Check sheet for the modelled part. Datum: model origin and axes. Units: mm. Face numbers are marked on the shaded views. A direction names the side the tool comes from. Coordinates: 2 decimals unless noted, no trailing zeros. Loops run counter-clockwise (first coordinate to the right, second up) from the corner with the lowest first, then second, coordinate; pieces in that order, holes last.
```python
from build123d import *

# Parameters (mm, degrees)
SKETCH1_W           = 46.99
SKETCH1_H           = 15.875
BOSS_EXTRUDE1_DEPTH = 21.59
SKETCH2_W           = 43.18
SKETCH2_H           = 12.7
SKETCH2_W_2         = 27.94
SKETCH2_H_2         = 1.5875
CUT_EXTRUDE1_DEPTH  = 20.0025
SKETCH3_R           = 9.525
BOSS_EXTRUDE2_DEPTH = 1.5875
FILLET1_R           = 6.35
FILLET2_R           = 1.27
SKETCH9_W           = 27.94
SKETCH9_H           = 1.5875
BOSS_EXTRUDE3_DEPTH = 7.62


with BuildPart() as part:
    # Sketch1 → Boss-Extrude1 (new body)
    with BuildSketch(Plane(origin=(0, 0, 0), x_dir=(1, 0, 0), z_dir=(0, 1, 0))):
        Rectangle(SKETCH1_W, SKETCH1_H)
    extrude(amount=BOSS_EXTRUDE1_DEPTH)

    # Sketch2 → Cut-Extrude1 (cut)
    with BuildSketch(Plane(origin=(0, 21.59, 0), x_dir=(1, 0, 0), z_dir=(0, 1, 0))):
        Rectangle(SKETCH2_W, SKETCH2_H)
        with Locations((0, -7.14375)):
            Rectangle(SKETCH2_W_2, SKETCH2_H_2)
    extrude(amount=-CUT_EXTRUDE1_DEPTH, mode=Mode.SUBTRACT)

    # Sketch3 → Boss-Extrude2 (add)
    with BuildSketch(Plane.XY.offset(-6.35)):
        with Locations((0, 21.59)):
            Circle(SKETCH3_R)
    extrude(amount=-BOSS_EXTRUDE2_DEPTH)

    # Sketch7 → CSK for #6 Flat Head Machine Screw (100)1 (revolve, cut)
    with BuildSketch(Plane(origin=(0, 21.59, -6.35), x_dir=(0, -1, 0), z_dir=(1, 0, 0))):
        Polygon((0, 0), (0, 1.5875), (1.89865, 1.5875), (1.89865, 1.380025208), (3.5433, 0), align=None)
    revolve(axis=Axis((0, 21.59, 0), (0, 0, -1)), mode=Mode.SUBTRACT)

    # Fillet1
    fillet1_edges = [part.edges().sort_by_distance(p)[0] for p in [
        (9.525, 21.59, -7.14375),
        (-9.525, 21.59, -7.14375),
    ]]
    fillet(fillet1_edges, radius=FILLET1_R)

    # Fillet2
    fillet2_edges = [part.edges().sort_by_distance(p)[0] for p in [
        (23.495, 10.795, 7.9375),
        (-23.495, 10.795, 7.9375),
    ]]
    fillet(fillet2_edges, radius=FILLET2_R)

    # Sketch9 → Boss-Extrude3 (add)
    with BuildSketch(Plane(origin=(0, 1.5875, 0), x_dir=(1, 0, 0), z_dir=(0, 1, 0))):
        with Locations((0, -7.14375)):
            Rectangle(SKETCH9_W, SKETCH9_H)
    extrude(amount=BOSS_EXTRUDE3_DEPTH)


solid = part.part
```
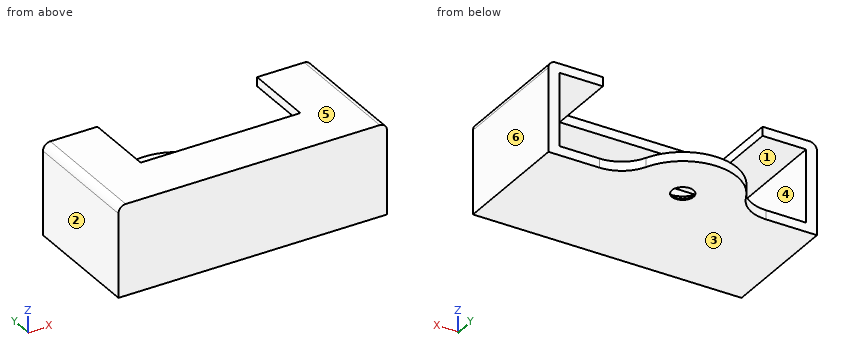
1) Set-up check for the marked faces 1 and 2: record each of +Z, -Z, +X, -X, +Y, -Y from which the full face is reachable in a straight line by a thin tool's end or side.
Answer sheet:
face 1: +Y
face 2: +Z, -Z, -X, +Y, -Y
2) Scan lines: line 1 (Z direction, x = 21, y = 13.5); line 2 (X direction, y = 15, z = 4) (3 decimals); line 3 (Z direction, x = 8.5, y = 16). Record each from-to range of solid material in increasing order.
Answer sheet:
line 1: z = -7.94 to -6.35, 6.35 to 7.94
line 2: x = -23.495 to -21.59, 21.59 to 23.495
line 3: z = -7.94 to -6.35
3) Depth check by flat-ended pin: pin 1 (3 mm diameter, centred on x = 1.5, z = 4, fed in from +Y); pin 2 (1.3 mm diameter, centred on x = 0.5, z = 7, fed in from +Y); pin 3 (0.5 mm diameter, centred on y = 16, z = 7, fed in from +X). Enter the tip coordinate at first touch or a pass-through.
Answer sheet:
pin 1: stops at y = 1.59
pin 2: stops at y = 9.21
pin 3: stops at x = 23.49
4) Section check C-C on z = -4.5. Enter the section's corners in (x, y) (1 decimal), plus the area to 3 significant figures.
Answer sheet:
outline: (-23.5, 0) - (23.5, 0) - (23.5, 21.6) - (21.6, 21.6) - (21.6, 1.6) - (-21.6, 1.6) - (-21.6, 21.6) - (-23.5, 21.6) - close
area: 151 mm2
5) Section check D-D on x = -19.5. Enter the section's corners in (y, z).
Answer sheet:
outline: (0, -7.94) - (21.59, -7.94) - (21.59, -6.35) - (1.59, -6.35) - (1.59, 6.35) - (21.59, 6.35) - (21.59, 7.94) - (0, 7.94) - close
6) Mould release check, pull along Z, two halves, no side actions. Record for the marked faces 3, 4, 5 and 6: +Z half, -Z half, draft (parallel to the pull), parting line (faces both ways), or undercut.
Answer sheet:
face 3: -Z half
face 4: undercut
face 5: +Z half
face 6: draft
